The model under review builds one solid part; all positions refer to its coordinate system, in mm. Face numbers are marked on the shaded views. A direction names the side the tool comes from. Round coordinates to 2 decimals unless told otherwise and drop trailing zeros. Order: outer loops, then holes, each group sorted by start corner. A loop starts at its lowest first (then second) coordinate and runs counter-clockwise, first axis right, second up.
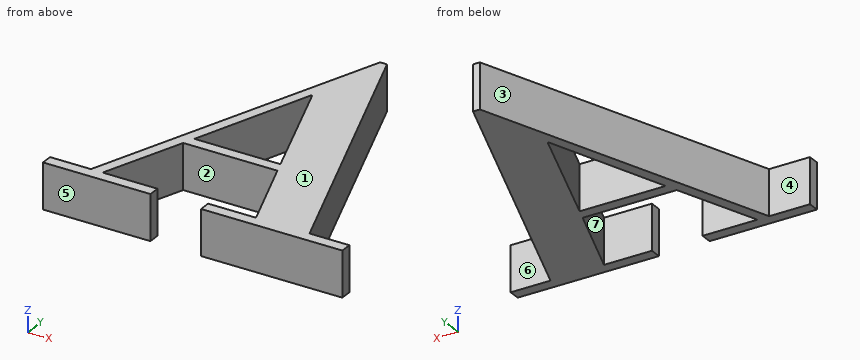
from build123d import *

# Parameters (mm, degrees)
F1_DEPTH = 45


with BuildPart() as f1:
    # F0 (on Top) → F1 (new body)
    with BuildSketch(Plane.XY):
        Polygon((-66.034691, -58.600819), (27.11419, -58.600819), (55.758373, -138.848471), (8.309083, -138.848471), (8.309083, -150), (148.032041, -150), (148.032041, -138.848471), (108.67285, -138.848471), (6.122862, 150), (-0.655503, 150), (-107.580103, -138.848471), (-148.032042, -138.848471), (-148.032042, -150), (-41.763672, -150), (-41.763672, -138.848471), (-95.990605, -138.848471), align=None)
        Polygon((23.178273, -47.44929), (-61.880509, -47.44929), (-19.023366, 69.970609), (-18.148157, 69.970609), align=None, mode=Mode.SUBTRACT)
    extrude(amount=F1_DEPTH)


solid = f1.part
(1) We need section B-B (x = -84). Give the boundary of the cut face in (y, z), and give its area (3 significant figures).
(2) We need section C-C (y = -112.5). Give the boundary of the cut face in (x, z), and give its area (3 significant figures).
(3) Clearance check with flat-ended pins moving along their axes: P1, Ø4, axis at y = -105, z = 19, coming from the -X side; P2, Ø0.7, axis at x = -18.5, z = 19.5, coming from the -Y side; P3, Ø1, axis at y = -4, z = 15.5, coming from the -X side. State where each tip first meets the part, or that it passes through.
(4) We need section D-D (x = -118.5). Give the boundary of the cut face in (y, z).
(5) The part is to be moulded in two halves that separate along X. For the marked faces 1, 2 and 3, say which applies: pulls with the +X half, pulls with the -X half, needs draft (parallel to the pull), parting line crosses it, or undercut.
(6) We need section A-A (z = 32). Give the boundary of the cut face in (x, y).
(7) Tool access review of the marked faces 4, 5, 6 and 7: name each direction out of +Z, -Z, +X, -X, +Y, -Y from which nothing blocks a thin tool from reaching the whole face with its end or side.
(8) To check wall thickness, follow L1, parallel to Y at x = -130, z = 37; L2, parallel to X at y = -40, z = 21; L3, parallel to X at y = -86.5, z = 39. State the ranges of each line that lie inside material, in increasing order.
Verdict:
1. outline: (-150, 0) - (-138.85, 0) - (-138.85, 45) - (-150, 45) - close; (-106.73, 0) - (-75.15, 0) - (-75.15, 45) - (-106.73, 45) - close
1. area: 1,920 mm2
2. outline: (-97.83, 0) - (-86.15, 0) - (-86.15, 45) - (-97.83, 45) - close; (46.35, 0) - (99.32, 0) - (99.32, 45) - (46.35, 45) - close
2. area: 2,910 mm2
3. P1: stops at x = -95.79
3. P2: stops at y = -58.6
3. P3: stops at x = -57.85
4. outline: (-150, 0) - (-138.85, 0) - (-138.85, 45) - (-150, 45) - close
5. face 1: needs draft
5. face 2: undercut
5. face 3: pulls with the -X half
6. outline: (-148.03, -150) - (-41.76, -150) - (-41.76, -138.85) - (-95.99, -138.85) - (-66.03, -58.6) - (27.11, -58.6) - (55.76, -138.85) - (8.31, -138.85) - (8.31, -150) - (148.03, -150) - (148.03, -138.85) - (108.67, -138.85) - (6.12, 150) - (-0.66, 150) - (-107.58, -138.85) - (-148.03, -138.85) - close; hole (-61.88, -47.45) - (23.18, -47.45) - (-18.15, 69.97) - (-19.02, 69.97) - close
7. face 4: +Z, -Z, -X, +Y
7. face 5: +Z, -Z, +X, -X, -Y
7. face 6: +Z, -Z, +X, +Y
7. face 7: +Z, -Z
8. L1: y = -150 to -138.85
8. L2: x = -70.99 to -59.16, 20.56 to 73.58
8. L3: x = -88.2 to -76.45, 37.07 to 90.09
